Read the model definition and answer for the solid it produces. Units are mm, in the model's axes. Give positions to 0.01 mm unless a question says otherwise; leave off trailing zeros. Loops run counter-clockwise (first coordinate to the right, second up) from the corner with the lowest first, then second, coordinate; pieces in that order, holes last. Notation, with made-up numbers: (48, 36) - (56, 36) arc R16 cw to (56, 55) - close; hole circle Ø3 at (29.5, 51). An arc over 180 degrees is marked (long way). Put each result on its own line as item: value. Start each with the question number.
1. Consider L1, parallel to X at y = 2.5, z = 48; L2, parallel to X at y = -0.5, z = 56; L3, parallel to X at y = 2.5, z = 67.5. Determine where each line is inside the solid, lowest interval first. Write a range as from..to.
2. A cutting plane is placed at A-A, the plane z = -69.85. Determine the outline of the cut face in (x, y) (1 decimal).
3. Given pin 1 Ø8 at (x, z) = (73.03, -29.65) entering from +Y (3 decimals); pin 2 Ø8 at (x, z) = (-40, 33.5) entering from -Y; pin 3 Ø6 at (x, z) = (-42.5, -3) entering from +Y, each flat-ended and moving along its own axis, determine where each tip first touches the part or whether it passes through.
4. A cutting plane is placed at D-D, the plane y = -1. Count the separate pieces of the cut face and the enclosed holes in it, plus the area to 3 significant figures.
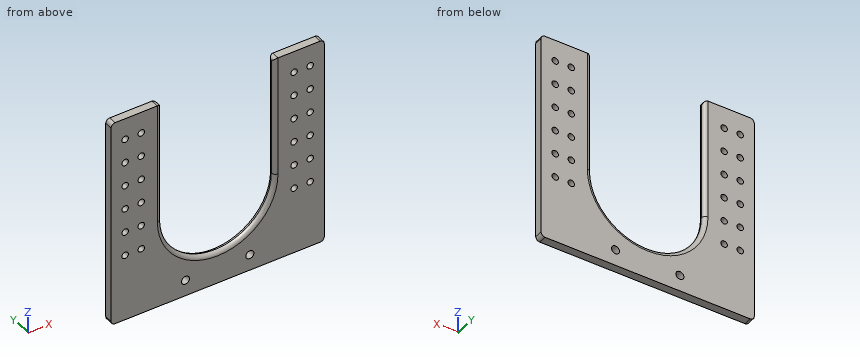
```python
from build123d import *

# Parameters (mm, degrees)
SKETCH1_W                        = 168.275
SKETCH1_H                        = 165.1
BOSS_EXTRUDE1_DEPTH              = 3.175
CUT_EXTRUDE1_REACH               = 120.042
SKETCH2_R                        = 44.45
F_1_4_0_25_DIAMETER_HOLE1_D      = 6.35
F_1_4_0_25_DIAMETER_HOLE1_DEPTH  = 25.4
F_1_4_0_25_DIAMETER_HOLE1_TIP    = 1.907732465
F_1_4_20_TAPPED_HOLE1_AT_2_COUNT = 2
F_1_4_20_TAPPED_HOLE1_AT_2_PITCH = 12.7
LPATTERN1_COUNT                  = 6
LPATTERN1_PITCH                  = 19.05
FILLET1_R                        = 3.175
FILLET2_R                        = 3.175


with BuildPart() as part:
    # Sketch1 → Boss-Extrude1 (new, symmetric)
    with BuildSketch(Plane(origin=(0, 0, 0), x_dir=(1, 0, 0), z_dir=(0, 1, 0))):
        Rectangle(SKETCH1_W, SKETCH1_H)
    extrude(amount=BOSS_EXTRUDE1_DEPTH, both=True)

    # Sketch2 → Cut-Extrude1 (cut, up to next)
    with BuildSketch(Plane(origin=(0, 3.175, 0), x_dir=(1, 0, 0), z_dir=(0, 1, 0)), mode=Mode.PRIVATE) as cut_extrude1_sk1:
        with Locations((0, 12.7)):
            Circle(SKETCH2_R)
    cut_extrude1_tool1 = extrude(cut_extrude1_sk1.sketch, amount=-CUT_EXTRUDE1_REACH, mode=Mode.PRIVATE) & part.part
    # Sketch2 → Cut-Extrude1 (cut, up to next)
    with BuildSketch(Plane(origin=(0, 3.175, 0), x_dir=(1, 0, 0), z_dir=(0, 1, 0)), mode=Mode.PRIVATE) as cut_extrude1_sk2:
        with BuildLine():
            Line((44.45, -82.55), (44.45, 12.7))
            ThreePointArc((44.45, 12.7), (0, -31.75), (-44.45, 12.7))
            Line((-44.45, 12.7), (-44.45, -82.55))
            Line((-44.45, -82.55), (44.45, -82.55))
        make_face()
    cut_extrude1_tool2 = extrude(cut_extrude1_sk2.sketch, amount=-CUT_EXTRUDE1_REACH, mode=Mode.PRIVATE) & part.part
    add(cut_extrude1_tool1.solids().sort_by_distance((0, 3.175, -12.7))[0], mode=Mode.SUBTRACT)
    add(cut_extrude1_tool2.solids().sort_by_distance((0, 3.175, 51.564855))[0], mode=Mode.SUBTRACT)

    # 1/4 (0.25) Diameter Hole1
    with Locations(Plane(origin=(0, 3.175, 0), x_dir=(1, 0, 0), z_dir=(0, 1, 0))):
        with Locations((-25.4, 69.85), (25.4, 69.85)):
            Hole(F_1_4_0_25_DIAMETER_HOLE1_D / 2, depth=F_1_4_0_25_DIAMETER_HOLE1_DEPTH)
            with Locations((0, 0, -(F_1_4_0_25_DIAMETER_HOLE1_DEPTH + F_1_4_0_25_DIAMETER_HOLE1_TIP / 2))):  # 118° drill point
                Cone(0, F_1_4_0_25_DIAMETER_HOLE1_D / 2, F_1_4_0_25_DIAMETER_HOLE1_TIP, mode=Mode.SUBTRACT)

    # Sketch10 → 1/4-20 Tapped Hole1 (revolve, cut)
    with BuildSketch(Plane(origin=(-73.025, 3.175, 65.603705108), x_dir=(0, 0, 1), z_dir=(1, 0, 0))):
        Polygon((0, 0), (0, 26.933816902), (2.5527, 25.4), (2.5527, 0), align=None)
    f_1_4_20_tapped_hole1 = revolve(axis=Axis((-73.025, 9.525, 65.603705108), (0, -1, 0)), mode=Mode.SUBTRACT)

    # 1/4-20 Tapped Hole1 at 2: 1/4-20 Tapped Hole1 ×2
    with Locations(*[(i * F_1_4_20_TAPPED_HOLE1_AT_2_PITCH, 0, 0) for i in range(1, F_1_4_20_TAPPED_HOLE1_AT_2_COUNT)]):
        add(f_1_4_20_tapped_hole1, mode=Mode.SUBTRACT)

    # LPattern1: 1/4-20 Tapped Hole1 ×6
    with Locations(*[(0, 0, -i * LPATTERN1_PITCH) for i in range(1, LPATTERN1_COUNT)]):
        add(f_1_4_20_tapped_hole1, mode=Mode.SUBTRACT)

    # LPattern1 copy 1 sketch → LPattern1 copy 1 (revolve, cut)
    with BuildSketch(Plane(origin=(-60.325, 3.175, 46.553705108), x_dir=(0, 0, 1), z_dir=(1, 0, 0))):
        Polygon((0, 0), (0, 26.933816902), (2.5527, 25.4), (2.5527, 0), align=None)
    revolve(axis=Axis((-60.325, 9.525, 46.553705108), (0, -1, 0)), mode=Mode.SUBTRACT)

    # LPattern1 copy 2 sketch → LPattern1 copy 2 (revolve, cut)
    with BuildSketch(Plane(origin=(-60.325, 3.175, 27.503705108), x_dir=(0, 0, 1), z_dir=(1, 0, 0))):
        Polygon((0, 0), (0, 26.933816902), (2.5527, 25.4), (2.5527, 0), align=None)
    revolve(axis=Axis((-60.325, 9.525, 27.503705108), (0, -1, 0)), mode=Mode.SUBTRACT)

    # LPattern1 copy 3 sketch → LPattern1 copy 3 (revolve, cut)
    with BuildSketch(Plane(origin=(-60.325, 3.175, 8.453705108), x_dir=(0, 0, 1), z_dir=(1, 0, 0))):
        Polygon((0, 0), (0, 26.933816902), (2.5527, 25.4), (2.5527, 0), align=None)
    revolve(axis=Axis((-60.325, 9.525, 8.453705108), (0, -1, 0)), mode=Mode.SUBTRACT)

    # LPattern1 copy 4 sketch → LPattern1 copy 4 (revolve, cut)
    with BuildSketch(Plane(origin=(-60.325, 3.175, -10.596294892), x_dir=(0, 0, 1), z_dir=(1, 0, 0))):
        Polygon((0, 0), (0, 26.933816902), (2.5527, 25.4), (2.5527, 0), align=None)
    revolve(axis=Axis((-60.325, 9.525, -10.596294892), (0, -1, 0)), mode=Mode.SUBTRACT)

    # LPattern1 copy 5 sketch → LPattern1 copy 5 (revolve, cut)
    with BuildSketch(Plane(origin=(-60.325, 3.175, -29.646294892), x_dir=(0, 0, 1), z_dir=(1, 0, 0))):
        Polygon((0, 0), (0, 26.933816902), (2.5527, 25.4), (2.5527, 0), align=None)
    revolve(axis=Axis((-60.325, 9.525, -29.646294892), (0, -1, 0)), mode=Mode.SUBTRACT)

    # Mirror1: 1/4-20 Tapped Hole1 across plane
    add(f_1_4_20_tapped_hole1.mirror(Plane(origin=(0, 0, 0), x_dir=(0, 0, 1), z_dir=(1, 0, 0))), mode=Mode.SUBTRACT)

    # Mirror1 copy 1 sketch → Mirror1 copy 1 (revolve, cut)
    with BuildSketch(Plane(origin=(60.325, 3.175, 65.603705108), x_dir=(0, 0, 1), z_dir=(-1, 0, 0))):
        Polygon((0, 0), (0, -26.933816902), (2.5527, -25.4), (2.5527, 0), align=None)
    revolve(axis=Axis((60.325, 9.525, 65.603705108), (0, 1, 0)), mode=Mode.SUBTRACT)

    # Mirror1 copy 2 sketch → Mirror1 copy 2 (revolve, cut)
    with BuildSketch(Plane(origin=(73.025, 3.175, 46.553705108), x_dir=(0, 0, 1), z_dir=(-1, 0, 0))):
        Polygon((0, 0), (0, -26.933816902), (2.5527, -25.4), (2.5527, 0), align=None)
    revolve(axis=Axis((73.025, 9.525, 46.553705108), (0, 1, 0)), mode=Mode.SUBTRACT)

    # Mirror1 copy 3 sketch → Mirror1 copy 3 (revolve, cut)
    with BuildSketch(Plane(origin=(73.025, 3.175, 27.503705108), x_dir=(0, 0, 1), z_dir=(-1, 0, 0))):
        Polygon((0, 0), (0, -26.933816902), (2.5527, -25.4), (2.5527, 0), align=None)
    revolve(axis=Axis((73.025, 9.525, 27.503705108), (0, 1, 0)), mode=Mode.SUBTRACT)

    # Mirror1 copy 4 sketch → Mirror1 copy 4 (revolve, cut)
    with BuildSketch(Plane(origin=(73.025, 3.175, 8.453705108), x_dir=(0, 0, 1), z_dir=(-1, 0, 0))):
        Polygon((0, 0), (0, -26.933816902), (2.5527, -25.4), (2.5527, 0), align=None)
    revolve(axis=Axis((73.025, 9.525, 8.453705108), (0, 1, 0)), mode=Mode.SUBTRACT)

    # Mirror1 copy 5 sketch → Mirror1 copy 5 (revolve, cut)
    with BuildSketch(Plane(origin=(73.025, 3.175, -10.596294892), x_dir=(0, 0, 1), z_dir=(-1, 0, 0))):
        Polygon((0, 0), (0, -26.933816902), (2.5527, -25.4), (2.5527, 0), align=None)
    revolve(axis=Axis((73.025, 9.525, -10.596294892), (0, 1, 0)), mode=Mode.SUBTRACT)

    # Mirror1 copy 6 sketch → Mirror1 copy 6 (revolve, cut)
    with BuildSketch(Plane(origin=(73.025, 3.175, -29.646294892), x_dir=(0, 0, 1), z_dir=(-1, 0, 0))):
        Polygon((0, 0), (0, -26.933816902), (2.5527, -25.4), (2.5527, 0), align=None)
    revolve(axis=Axis((73.025, 9.525, -29.646294892), (0, 1, 0)), mode=Mode.SUBTRACT)

    # Mirror1 copy 7 sketch → Mirror1 copy 7 (revolve, cut)
    with BuildSketch(Plane(origin=(60.325, 3.175, 46.553705108), x_dir=(0, 0, 1), z_dir=(-1, 0, 0))):
        Polygon((0, 0), (0, -26.933816902), (2.5527, -25.4), (2.5527, 0), align=None)
    revolve(axis=Axis((60.325, 9.525, 46.553705108), (0, 1, 0)), mode=Mode.SUBTRACT)

    # Mirror1 copy 8 sketch → Mirror1 copy 8 (revolve, cut)
    with BuildSketch(Plane(origin=(60.325, 3.175, 27.503705108), x_dir=(0, 0, 1), z_dir=(-1, 0, 0))):
        Polygon((0, 0), (0, -26.933816902), (2.5527, -25.4), (2.5527, 0), align=None)
    revolve(axis=Axis((60.325, 9.525, 27.503705108), (0, 1, 0)), mode=Mode.SUBTRACT)

    # Mirror1 copy 9 sketch → Mirror1 copy 9 (revolve, cut)
    with BuildSketch(Plane(origin=(60.325, 3.175, 8.453705108), x_dir=(0, 0, 1), z_dir=(-1, 0, 0))):
        Polygon((0, 0), (0, -26.933816902), (2.5527, -25.4), (2.5527, 0), align=None)
    revolve(axis=Axis((60.325, 9.525, 8.453705108), (0, 1, 0)), mode=Mode.SUBTRACT)

    # Mirror1 copy 10 sketch → Mirror1 copy 10 (revolve, cut)
    with BuildSketch(Plane(origin=(60.325, 3.175, -10.596294892), x_dir=(0, 0, 1), z_dir=(-1, 0, 0))):
        Polygon((0, 0), (0, -26.933816902), (2.5527, -25.4), (2.5527, 0), align=None)
    revolve(axis=Axis((60.325, 9.525, -10.596294892), (0, 1, 0)), mode=Mode.SUBTRACT)

    # Mirror1 copy 11 sketch → Mirror1 copy 11 (revolve, cut)
    with BuildSketch(Plane(origin=(60.325, 3.175, -29.646294892), x_dir=(0, 0, 1), z_dir=(-1, 0, 0))):
        Polygon((0, 0), (0, -26.933816902), (2.5527, -25.4), (2.5527, 0), align=None)
    revolve(axis=Axis((60.325, 9.525, -29.646294892), (0, 1, 0)), mode=Mode.SUBTRACT)

    # Fillet1
    fillet1_edges = [part.edges().sort_by_distance(p)[0] for p in [
        (-44.45, -3.175, 34.925),
        (0, -3.175, -57.15),
        (-44.45, 3.175, 34.925),
        (0, 3.175, -57.15),
        (44.45, -3.175, 34.925),
        (44.45, 3.175, 34.925),
        (84.1375, 0, 82.55),
        (44.45, 0, 82.55),
        (-84.1375, 0, 82.55),
        (-44.45, 0, 82.55),
    ]]
    fillet(fillet1_edges, radius=FILLET1_R - 0.0001)  # a hair under: the kernel refuses the full size

    # Fillet2
    fillet2_edges = [part.edges().sort_by_distance(p)[0] for p in [
        (84.1375, 0, -82.55),
        (-84.1375, 0, -82.55),
    ]]
    fillet(fillet2_edges, radius=FILLET2_R)


solid = part.part
```
Return value:
1. L1: x = -84.14..-75.13, -70.92..-62.43, -58.22..-45.67, 45.67..58.22, 62.43..70.92, 75.13..84.14
1. L2: x = -84.14..-44.49, 44.49..84.14
1. L3: x = -84.14..-74.73, -71.32..-62.03, -58.62..-45.67, 45.67..58.62, 62.03..71.32, 74.73..84.14
2. outline: (-84.1, -3.2) - (-28.6, -3.2) - (-28.6, 3.2) - (-84.1, 3.2) - close; (-22.2, -3.2) - (22.2, -3.2) - (22.2, 3.2) - (-22.2, 3.2) - close; (28.6, -3.2) - (84.1, -3.2) - (84.1, 3.2) - (28.6, 3.2) - close
3. pin 1: stops at y = 3.175
3. pin 2: passes through
3. pin 3: stops at y = 2.36
4. separate pieces: 1
4. enclosed holes: 26
4. area: 15,600 mm2
